Check sheet for the modelled part. Datum: model origin and axes. Units: mm. Face numbers are marked on the shaded views. A direction names the side the tool comes from. Round coordinates to 2 decimals unless told otherwise and drop trailing zeros. Write each loop counter-clockwise with the first axis right and the second up, starting at its lowest first coordinate (ties: lowest second). Pieces come first, ordered by that corner, then holes. Notation, with made-up numbers: M 47.25,32 L 104.25,32 A20 cw 104.25,37 Z; hole C 56.25,-5.5 d9. An arc over 180 degrees is marked long. Answer in a Markdown table with one row per item.
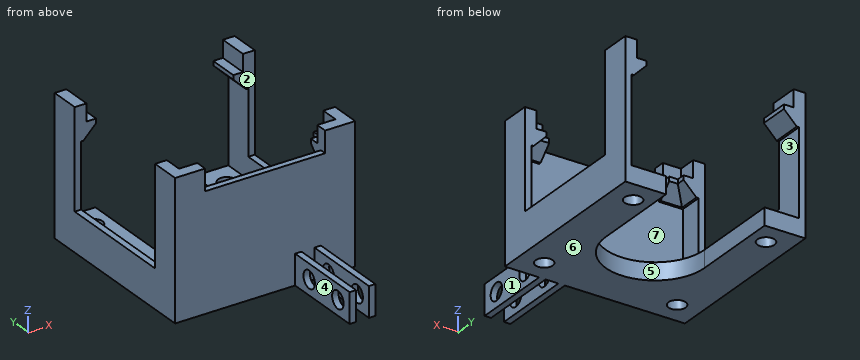
```python
from build123d import *

# Parameters (mm, degrees)
F0_R      = 2
F0_W      = 1.5
F0_H      = 28
F0_W_2    = 28
F0_H_2    = 1.5
F0_W_3    = 8
F1_DEPTH  = 4
F2_DEPTH  = 23
F3_DEPTH  = 5
F4_W      = 2.75
F4_H      = 7
F5_DEPTH  = 5
F4_W_2    = 2.25
F6_DEPTH  = 1
F7_DEPTH  = 3
F8_SIZE   = 3
F9_W      = 1.5
F9_H      = 7
F10_DEPTH = 19
F11_R     = 2
F12_DEPTH = 14.001


# Not quite as in the source:
# - a feature names something its author has since deleted; it is built from what else it names


with BuildPart() as f1:
    # F0 (on Top) → F1 (new body)
    with BuildSketch(Plane.XY):
        with BuildLine():
            Line((-11.5, 19.5), (-19.5, 19.5))
            Line((-19.5, 19.5), (-19.5, 14))
            Line((-19.5, 14), (-19.5, -14))
            Line((-19.5, -14), (-19.5, -19.5))
            Line((-19.5, -19.5), (-14, -19.5))
            Line((-14, -19.5), (14, -19.5))
            Line((14, -19.5), (19.5, -19.5))
            Line((19.5, -19.5), (19.5, -14))
            Line((19.5, -14), (19.5, 14))
            Line((19.5, 14), (19.5, 19.5))
            Line((19.5, 19.5), (11.5, 19.5))
            Line((11.5, 19.5), (11.5, 0))
            ThreePointArc((11.5, 0), (0, -11.5), (-11.5, 0))
            Line((-11.5, 0), (-11.5, 19.5))
        make_face()
        with Locations((-15.5, -15.5)):
            Circle(F0_R, mode=Mode.SUBTRACT)
        with Locations((15.5, -15.5)):
            Circle(F0_R, mode=Mode.SUBTRACT)
        with Locations((-15.5, 15.5)):
            Circle(F0_R, mode=Mode.SUBTRACT)
        with Locations((15.5, 15.5)):
            Circle(F0_R, mode=Mode.SUBTRACT)
        with Locations((-20.25, 0)):
            Rectangle(F0_W, F0_H)
        Polygon((19.5, 21), (19.5, 19.5), (19.5, 14), (21, 14), (21, 21), align=None)
        Polygon((21, -14), (19.5, -14), (19.5, -19.5), (14, -19.5), (14, -21), (21, -21), align=None)
        Polygon((-19.5, -19.5), (-19.5, -14), (-21, -14), (-21, -21), (-14, -21), (-14, -19.5), align=None)
        Polygon((-19.5, 14), (-19.5, 19.5), (-19.5, 21), (-21, 21), (-21, 14), align=None)
        with Locations((20.25, 0)):
            Rectangle(F0_W, F0_H)
        with Locations((0, -20.25)):
            Rectangle(F0_W_2, F0_H_2)
        with Locations((-15.5, 20.25)):
            Rectangle(F0_W_3, F0_H_2)
        with Locations((15.5, 20.25)):
            Rectangle(F0_W_3, F0_H_2)
    extrude(amount=-F1_DEPTH)

    # F0 (on Top) → F2 (join)
    with BuildSketch(Plane.XY):
        Polygon((-19.5, -19.5), (-19.5, -14), (-21, -14), (-21, -21), (-14, -21), (-14, -19.5), align=None)
        Polygon((21, -14), (19.5, -14), (19.5, -19.5), (14, -19.5), (14, -21), (21, -21), align=None)
        Polygon((-19.5, 14), (-19.5, 19.5), (-19.5, 21), (-21, 21), (-21, 14), align=None)
        Polygon((19.5, 21), (19.5, 19.5), (19.5, 14), (21, 14), (21, 21), align=None)
        with Locations((0, -20.25)):
            Rectangle(F0_W_2, F0_H_2)
    extrude(amount=F2_DEPTH)

    # F0 (on Top) → F3 (join)
    with BuildSketch(Plane.XY):
        with Locations((20.25, 0)):
            Rectangle(F0_W, F0_H)
        with Locations((-20.25, 0)):
            Rectangle(F0_W, F0_H)
    extrude(amount=F3_DEPTH)

    # F4 (on face) → F5 (join)
    with BuildSketch(Plane.XY.offset(23)):
        with Locations((19.625, 17.5)):
            Rectangle(F4_W, F4_H)
        Polygon((14, -19.5), (14, -21), (21, -21), (21, -14), (19.5, -14), (19.5, -19.5), align=None)
        Polygon((-19.5, -19.5), (-21, -21), (-14, -21), (-14, -19.5), align=None)
        Polygon((-18.25, -18.25), (-19.5, -19.5), (-14, -19.5), (-14, -18.25), align=None)
        Polygon((-18.25, -14), (-19.5, -14), (-19.5, -19.5), (-18.25, -18.25), align=None)
        Polygon((-19.5, -14), (-21, -14), (-21, -21), (-19.5, -19.5), align=None)
        with Locations((-19.625, 17.5)):
            Rectangle(F4_W, F4_H)
        Polygon((14, -18.25), (14, -19.5), (19.5, -19.5), (19.5, -14), (18.25, -14), (18.25, -18.25), align=None)
    extrude(amount=F5_DEPTH)

    # F4 (on face) → F6 (join)
    with BuildSketch(Plane.XY.offset(23)):
        with Locations((17.125, 17.5)):
            Rectangle(F4_W_2, F4_H)
        Polygon((14, -16), (14, -18.25), (18.25, -18.25), (18.25, -14), (16, -14), (16, -16), align=None)
        Polygon((-16, -16), (-18.25, -18.25), (-14, -18.25), (-14, -16), align=None)
        Polygon((-16, -14), (-18.25, -14), (-18.25, -18.25), (-16, -16), align=None)
        with Locations((-17.125, 17.5)):
            Rectangle(F4_W_2, F4_H)
    extrude(amount=F6_DEPTH)

    # F7 (add): faces of the model
    f7_faces = [f1.faces().sort_by_distance(p)[0] for p in [
        (17.75, 17.5, 23),
        (17.0166666667, -17.0166666667, 23),
        (-17.0166666667, -17.0166666667, 23),
        (-17.75, 17.5, 23),
    ]]
    extrude(f7_faces, amount=F7_DEPTH)

    # F8
    f8_edges = [f1.edges().sort_by_distance(p)[0] for p in [
        (16, 17.5, 20),
        (15, -16, 20),
        (16, -15, 20),
        (-15, -16, 20),
        (-16, -15, 20),
        (-16, 17.5, 20),
    ]]
    chamfer(f8_edges, length=F8_SIZE)

    # F9 (on face) → F10 (join)
    with BuildSketch(Plane.XZ.offset(21)):
        with Locations((7.75, -0.5)):
            Rectangle(F9_W, F9_H)
        with Locations((12.25, -0.5)):
            Rectangle(F9_W, F9_H)
    extrude(amount=F10_DEPTH)

    # F11 (on face) → F12 (cut, through all)
    with BuildSketch(Plane(origin=(7, 0, 0), x_dir=(0, -1, 0), z_dir=(-1, 0, 0))):
        with Locations((25.9, -0.5)):
            Circle(F11_R)
        with Locations((35.9, -0.5)):
            Circle(F11_R)
    extrude(amount=-F12_DEPTH, mode=Mode.SUBTRACT)


solid = f1.part
```
1. Section check C-C, the plane y = 15.5. Count the separate pieces of the cut face and the enclosed holes in it, and give its area (3 significant figures).
Found:
| item | result |
|---|---|
| separate pieces | 4 |
| enclosed holes | 0 |
| area | 157 mm2 |
2. Scan lines: L1, parallel to Y at x = -15.5, z = -2.3; L2, parallel to X at y = -19.5, z = 24.5; L3, parallel to Z at x = 12.15, y = -25.9. Record each from-to range of solid material in increasing order.
Found:
| item | result |
|---|---|
| L1 | y = -21 to -17.5, -13.5 to 13.5, 17.5 to 21 |
| L2 | x = -21 to -14, 14 to 21 |
| L3 | z = -4 to -2.5, 1.5 to 3 |
3. Draft check along Z on the marked faces 5, 6 and 7. Enter one of: +Z half, -Z half, draft (parallel to the pull), parting line (faces both ways), or undercut.
Found:
| item | result |
|---|---|
| face 5 | draft |
| face 6 | -Z half |
| face 7 | undercut |
4. Section check D-D, the plane z = 6.5. Record the cut outline in (x, y), and give its area (4 significant figures).
Found:
| item | result |
|---|---|
| outline | M -21,-21 L 21,-21 L 21,-14 L 19.5,-14 L 19.5,-19.5 L -19.5,-19.5 L -19.5,-14 L -21,-14 Z; M -21,14 L -19.5,14 L -19.5,21 L -21,21 Z; M 19.5,14 L 21,14 L 21,21 L 19.5,21 Z |
| area | 100.5 mm2 |
5. Go/stop test with flat-tipped pins: pin 1 (2 mm diameter, centred on y = -33.5, z = -1.5, fed in from -X); pin 2 (0.7 mm diameter, centred on x = 16.5, y = 17.5, fed in from +Z); pin 3 (1.5 mm diameter, centred on x = -17.5, z = 21.5, fed in from -Y). Record where each tip stops, or that it passes through.
Found:
| item | result |
|---|---|
| pin 1 | stops at x = 7 |
| pin 2 | stops at z = 24 |
| pin 3 | stops at y = -21 |
6. Section check A-A, the plane y = -33. Record the cut outline in (x, z), and give its area (3 significant figures).
Found:
| item | result |
|---|---|
| outline | M 7,-4 L 8.5,-4 L 8.5,3 L 7,3 Z; M 11.5,-4 L 13,-4 L 13,3 L 11.5,3 Z |
| area | 21.0 mm2 |
7. Access from +Z, -Z, +X, -X, +Y, -Y to the whole of each face (thin tool, end or side, straight path). Record for the marked faces 1, 2, 3 and 4.
Found:
| item | result |
|---|---|
| face 1 | +Z, -Z, +X, -Y |
| face 2 | +Z, +X, -X |
| face 3 | +Y |
| face 4 | +Z, -Z, -X, -Y |
8. Section check B-B, the plane z = 21.5. Record the cut outline in (x, y), and give its area (4 significant figures).
Found:
| item | result |
|---|---|
| outline | M -21,-21 L 21,-21 L 21,-14 L 17.5,-14 L 17.5,-17.5 L 14,-17.5 L 14,-19.5 L -14,-19.5 L -14,-17.5 L -17.5,-17.5 L -17.5,-14 L -21,-14 Z; M -21,14 L -17.5,14 L -17.5,21 L -21,21 Z; M 17.5,14 L 21,14 L 21,21 L 17.5,21 Z |
| area | 164.5 mm2 |
